For this review, take the finished solid that the model builds, in its own axes (mm). Face numbers are marked on the shaded views. A direction names the side the tool comes from. Coordinates: 2 decimals unless noted, no trailing zeros. Order: outer loops, then holes, each group sorted by start corner. A loop starts at its lowest first (then second) coordinate and runs counter-clockwise, first axis right, second up.
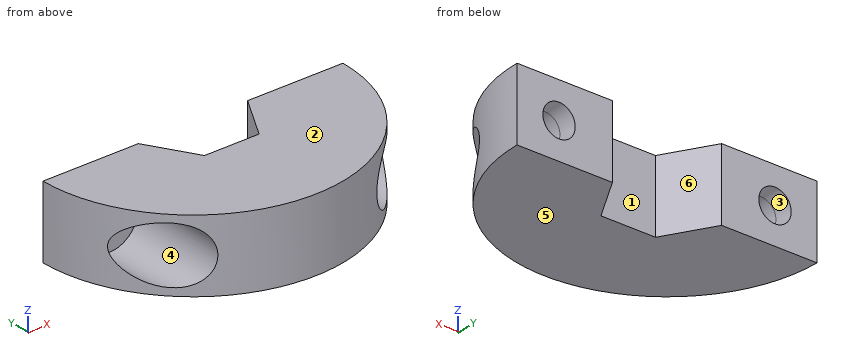
from build123d import *

# Parameters (mm, degrees)
BOSS_EXTRUDE1_DEPTH                          = 12
SKETCH2_R                                    = 4.75
CUT_EXTRUDE1_DEPTH                           = 35
SKETCH3_R                                    = 2.05
CUT_EXTRUDE2_DEPTH                           = 35
CUT_EXTRUDE3_DEPTH                           = 20
CSK_FOR_M3_CROSS_COUNTERSUNK_HEAD_SC_2_COUNT = 2
CSK_FOR_M3_CROSS_COUNTERSUNK_HEAD_SC_2_PITCH = 36


with BuildPart() as part:
    # Sketch1 → Boss-Extrude1 (new body)
    with BuildSketch(Plane.XY):
        with BuildLine():
            Line((-9.1, 0), (-25, 0))
            ThreePointArc((-25, 0), (0, -25), (25, 0))
            Line((25, 0), (9.211282306, 0))
            Line((9.211282306, 0), (9.1, 0))
            Line((9.1, 0), (-9.1, 0))
        make_face()
    extrude(amount=BOSS_EXTRUDE1_DEPTH)

    # Sketch2 → Cut-Extrude1 (cut)
    with BuildSketch(Plane(origin=(0, -40, 0), x_dir=(1, 0, 0), z_dir=(0, 1, 0))):
        with Locations((18, -6)):
            Circle(SKETCH2_R)
        with Locations((-18, -6)):
            Circle(SKETCH2_R)
    extrude(amount=CUT_EXTRUDE1_DEPTH, mode=Mode.SUBTRACT)

    # Sketch3 → Cut-Extrude2 (cut)
    with BuildSketch(Plane.XZ.offset(5)):
        with Locations((18, 6)):
            Circle(SKETCH3_R)
        with Locations((-18, 6)):
            Circle(SKETCH3_R)
    extrude(amount=-CUT_EXTRUDE2_DEPTH, mode=Mode.SUBTRACT)

    # Sketch4 → Cut-Extrude3 (cut)
    with BuildSketch(Plane.XY.offset(12)):
        Polygon((9.1, 0), (4.55, 7.880831174), (-4.55, 7.880831174), (-9.1, 0), (-4.55, -7.880831174), (4.55, -7.880831174), align=None)
    extrude(amount=-CUT_EXTRUDE3_DEPTH, mode=Mode.SUBTRACT)

    # Sketch5 → CSK for M3 Cross Countersunk Head Screw1 (revolve, cut)
    with BuildSketch(Plane(origin=(-18, 0, 6), x_dir=(0, 0, 1), z_dir=(1, 0, 0))):
        Polygon((0, 0), (0, 25), (2.5, 25), (2.5, 2.860133251), (2.7, 0), align=None)
    csk_for_m3_cross_countersunk_head_screw1 = revolve(axis=Axis((-18, 6.35, 6), (0, -1, 0)), mode=Mode.SUBTRACT)

    # CSK for M3 Cross Countersunk Head Sc 2: CSK for M3 Cross Countersunk Head Screw1 ×2
    with Locations(*[(i * CSK_FOR_M3_CROSS_COUNTERSUNK_HEAD_SC_2_PITCH, 0, 0) for i in range(1, CSK_FOR_M3_CROSS_COUNTERSUNK_HEAD_SC_2_COUNT)]):
        add(csk_for_m3_cross_countersunk_head_screw1, mode=Mode.SUBTRACT)


solid = part.part
1. To check wall thickness, follow L1, parallel to X at y = -2, z = 5; L2, parallel to X at y = -4.5, z = 7.75; L3, parallel to Z at x = -18, y = -16. State the ranges of each line that lie inside material, in increasing order.
Answer below:
L1: x = -24.92 to -20.36, -15.64 to -7.95, 7.95 to 15.64, 20.36 to 24.92
L2: x = -24.59 to -19.79, -16.21 to -6.5, 6.5 to 16.21, 19.79 to 24.59
L3: z = 0 to 1.25, 10.75 to 12
2. Take a section at A-A, the plane z = 6. Give the boundary of the cut face in (x, y).
Answer below:
outline: (-25, 0) arc R25 ccw to (-22.75, -10.37) - (-22.75, -5) - (-20.5, -5) - (-20.5, -2.86) - (-20.7, 0) - close; (-15.5, -5) - (-13.25, -5) - (-13.25, -21.2) arc R25 ccw to (13.25, -21.2) - (13.25, -5) - (15.5, -5) - (15.5, -2.86) - (15.3, 0) - (9.1, 0) - (4.55, -7.88) - (-4.55, -7.88) - (-9.1, 0) - (-15.3, 0) - (-15.5, -2.86) - close; (20.5, -5) - (22.75, -5) - (22.75, -10.37) arc R25 ccw to (25, 0) - (20.7, 0) - (20.5, -2.86) - close
3. Take a section at B-B, the plane x = 18. Give the boundary of the cut face in (y, z), plus the area to 3 significant figures.
Answer below:
outline: (-17.35, 0) - (0, 0) - (0, 3.3) - (-2.86, 3.5) - (-5, 3.5) - (-5, 1.25) - (-17.35, 1.25) - close; (-17.35, 10.75) - (-5, 10.75) - (-5, 8.5) - (-2.86, 8.5) - (0, 8.7) - (0, 12) - (-17.35, 12) - close
area: 65.3 mm2
4. Take a section at D-D, the plane z = 2.25. Give the boundary of the cut face in (x, y), plus the area to 3 significant figures.
Answer below:
outline: (-25, 0) arc R25 ccw to (-20.92, -13.69) - (-20.92, -5) - (-15.08, -5) - (-15.08, -19.94) arc R25 ccw to (15.08, -19.94) - (15.08, -5) - (20.92, -5) - (20.92, -13.69) arc R25 ccw to (25, 0) - (9.1, 0) - (4.55, -7.88) - (-4.55, -7.88) - (-9.1, 0) - close
area: 732 mm2
5. The part is to be moulded in two halves that separate along Z. For the marked faces 1, 2 and 3, say which applies: +Z half, -Z half, draft (parallel to the pull), parting line (faces both ways), or undercut.
Answer below:
face 1: draft
face 2: +Z half
face 3: undercut
6. Clearance check with flat-ended pins moving along their axes: pin 1 Ø4 at (x, z) = (18, 6) entering from +Y (1 decimal); pin 2 Ø2 at (y, z) = (-4, 4) entering from +X; pin 3 Ø3 at (x, z) = (16.5, 7) entering from -Y; pin 4 Ø5 at (x, z) = (9.5, 9) entering from -Y. State where each tip first meets the part, or that it passes through.
Answer below:
pin 1: passes through
pin 2: stops at x = 24.82
pin 3: stops at y = -5
pin 4: stops at y = -24
7. Machinability: for the marked faces 4, 5 and 6, which of the approach directions +Z, -Z, +X, -X, +Y, -Y give a long, thin tool a straight path to every point of the face, cutting with its end or side? Answer none if there is none.
Answer below:
face 4: -Y
face 5: -Z, +X, -X, +Y, -Y
face 6: +Z, -Z, +Y
8. Take a section at C-C, the plane y = -8.5. Give the boundary of the cut face in (x, z).
Answer below:
outline: (-23.51, 0) - (23.51, 0) - (23.51, 12) - (-23.51, 12) - close; hole circle Ø9.5 at (-18, 6); hole circle Ø9.5 at (18, 6)
